from build123d import *

# Parameters (mm, degrees)
SKETCH1_R           = 7
SKETCH1_R_2         = 4
SKETCH1_R_3         = 17.5
BOSS_EXTRUDE1_DEPTH = 10
SKETCH4_R           = 4
SKETCH4_R_2         = 8
SKETCH4_R_3         = 16
CUT_EXTRUDE1_DEPTH  = 11


with BuildPart() as part:
    # Sketch1 → Boss-Extrude1 (new body)
    with BuildSketch(Plane.XY):
        with BuildLine():
            ThreePointArc((1.572195793, 94.986989637), (-94.380567411, -10.83090463), (23.048944019, -92.161522229))
            ThreePointArc((23.048944019, -92.161522229), (83.617990825, -93.079348945), (135.711425994, -123.994164958))
            ThreePointArc((135.711425994, -123.994164958), (165.350102595, -122.820856068), (161.225161537, -93.447183066))
            ThreePointArc((161.225161537, -93.447183066), (106.014165413, 10.833093568), (161.441107802, 114.998751274))
            ThreePointArc((161.441107802, 114.998751274), (165.454566443, 126.056147345), (156.171848547, 133.281450563))
            ThreePointArc((156.171848547, 133.281450563), (103.433194213, 127.791254655), (54.122076862, 108.299676532))
            ThreePointArc((54.122076862, 108.299676532), (28.73316338, 98.145871106), (1.572195793, 94.986989637))
        make_face()
        with Locations((66.321036094, 102.089205288)):
            Circle(SKETCH1_R, mode=Mode.SUBTRACT)
        with Locations((155.845687485, 123.28677103)):
            Circle(SKETCH1_R, mode=Mode.SUBTRACT)
        with Locations((150, -110)):
            Circle(SKETCH1_R, mode=Mode.SUBTRACT)
        with Locations((0, 74.6)):
            Circle(SKETCH1_R_2, mode=Mode.SUBTRACT)
        with Locations((74.6, 0)):
            Circle(SKETCH1_R_2, mode=Mode.SUBTRACT)
        with Locations((0, -74.6)):
            Circle(SKETCH1_R_2, mode=Mode.SUBTRACT)
        with Locations((-74.6, 0)):
            Circle(SKETCH1_R_2, mode=Mode.SUBTRACT)
        Circle(SKETCH1_R_3, mode=Mode.SUBTRACT)
    extrude(amount=BOSS_EXTRUDE1_DEPTH)

    # Sketch4 → Cut-Extrude1 (cut, through all)
    with BuildSketch(Plane.XY.offset(10)):
        with Locations((129.839875104, -95.215908409)):
            Circle(SKETCH4_R)
        with Locations((105.647725228, -77.4749985)):
            Circle(SKETCH4_R_2)
        with Locations((69.359500414, -50.863633637)):
            Circle(SKETCH4_R_3)
    extrude(amount=-CUT_EXTRUDE1_DEPTH, mode=Mode.SUBTRACT)


solid = part.part
Can you work these out from the model? Positions are in its coordinate system, mm. Coordinates: 2 decimals unless noted, no trailing zeros. Write each loop counter-clockwise with the first axis right and the second up, starting at its lowest first coordinate (ties: lowest second). Pieces come first, ordered by that corner, then holes. Notation, with made-up numbers: (63, 53.5) -> (117, 53.5) arc R13 ccw to (117, 72.5) -> close; hole circle Ø2 at (24.25, 32.5). An arc over 180 degrees is marked (long way). Answer as CSV lines item,"result".
1) If we section it at C-C on y = 0: Please give me the cut outline in (x, z).
Check result:
outline,"(-95, 0) -> (-78.6, 0) -> (-78.6, 10) -> (-95, 10) -> close; (-70.6, 0) -> (-17.5, 0) -> (-17.5, 10) -> (-70.6, 10) -> close; (17.5, 0) -> (70.6, 0) -> (70.6, 10) -> (17.5, 10) -> close; (78.6, 0) -> (106.47, 0) -> (106.47, 10) -> (78.6, 10) -> close"
2) If we section it at A-A on y = -110: Please give me the cut outline in (x, z).
Check result:
outline,"(119.23, 0) -> (143, 0) -> (143, 10) -> (119.23, 10) -> close; (157, 0) -> (170, 0) -> (170, 10) -> (157, 10) -> close"
3) If I drill on line 1 (Y direction, x = 131, z = 6.25); line 2 (Y direction, x = 144.5, z = 2.5); line 3 (X direction, y = -62, z = 4.5), over which ranges is the centre line in solid material (lowest first)? Write a range as from..to.
Check result:
line 1,"-119.44..-99.04, -91.39..-64.56, 85.96..132.48"
line 2,"-129.23..-114.33, -105.67..-79.88, 101.28..133.31"
line 3,"-71.98..57.87, 80.85..129.14"
4) If we mould it in two halves opening along Y, with no side actions, what happens to faces 1 (the cylindrical face through (104.157, 127.967, 4.93)), 2 (the cylindrical face through (113.038, -80.539, 5.07)), 3 (the cylindrical face through (-94.61, -8.58, 4.93))? For each: +Y half, -Y half, draft (parallel to the pull), parting line (faces both ways), or undercut.
Check result:
face 1,"+Y half"
face 2,"undercut"
face 3,"parting line"
5) If we section it at D-D on z = 4.25: Count the separate pieces of the cut face and the enclosed holes in it, then the cut area to 3 significant figures.
Check result:
separate pieces,"1"
enclosed holes,"11"
area,"38,900 mm²"
6) If we section it at B-B on x = 130: Please give me the cut outline in (y, z).
Check result:
outline,"(-118.54, 0) -> (-99.21, 0) -> (-99.21, 10) -> (-118.54, 10) -> close; (-91.22, 0) -> (-63.2, 0) -> (-63.2, 10) -> (-91.22, 10) -> close; (84.6, 0) -> (132.38, 0) -> (132.38, 10) -> (84.6, 10) -> close"
7) Will these pins go through, and if not, where does the flat tip stop? P1, Ø7, axis at x = 0, y = -74.6, coming from the +Z side; P2, Ø3, axis at x = 82, z = 6.5, coming from the -Y side; P3, Ø2, axis at x = -7.5, z = 2.5, coming from the +Y side; P4, Ø3, axis at y = 8.5, z = 3.5, coming from the -X side.
Check result:
P1,"through"
P2,"y = -93.05"
P3,"y = 94.78"
P4,"x = -94.74"
